```python
from build123d import *

# Parameters (mm, degrees)
F0_W     = 30
F0_H     = 20
F1_DEPTH = 7
F2_R     = 1.25
F3_DEPTH = 4
F4_W     = 30
F4_H     = 9
F5_DEPTH = 4


with BuildPart() as f1:
    # F0 (on Top) → F1 (new body)
    with BuildSketch(Plane.XY):
        Rectangle(F0_W, F0_H)
    extrude(amount=F1_DEPTH)

    # F2 (on face) → F3 (cut)
    with BuildSketch(Plane.XY.offset(7)):
        with Locations((5, 7.5)):
            Circle(F2_R)
        with Locations((-5, 7.5)):
            Circle(F2_R)
        with Locations((-5, -7.5)):
            Circle(F2_R)
        with Locations((5, -7.5)):
            Circle(F2_R)
    extrude(amount=-F3_DEPTH, mode=Mode.SUBTRACT)

    # F4 (on face) → F5 (cut)
    with BuildSketch(Plane(origin=(0, 0, 0), x_dir=(1, 0, 0), z_dir=(0, 0, -1))):
        Rectangle(F4_W, F4_H)
    extrude(amount=-F5_DEPTH, mode=Mode.SUBTRACT)


solid = f1.part
```
The listing builds one solid part. Answer for the finished solid, in the listing's coordinates (mm). A direction names the side the tool comes from. Coordinates: 2 decimals unless noted, no trailing zeros. Loops run counter-clockwise (first coordinate to the right, second up) from the corner with the lowest first, then second, coordinate; pieces in that order, holes last. Notation, with made-up numbers: (30.5, -15) -> (86.5, -15) arc R18 ccw to (86.5, -9) -> close; hole circle Ø9 at (-35.5, 47.5). An arc over 180 degrees is marked (long way). Return JSON: item names as keys, results as strings. Group by question number.
(1) Find the intervals of material crossed by probe 1 along Y at (x, z) = (5, 5.5); probe 2 along Y at (x, z) = (4.5, 6); probe 3 along Y at (x, z) = (5, 3.8), in increasing order. Write a range as from..to.
(2) Given pin 1 Ø0.8 at (x, y) = (-4.5, 7.5) entering from +Z; pin 2 Ø1 at (x, y) = (8.5, -1) entering from -Z, each flat-ended and moving along its own axis, determine where each tip first touches the part or whether it passes through.
(3) A cutting plane is placed at A-A on z = 5.25. Write down the section's boundary in (x, y).
(4) A cutting plane is placed at C-C on x = 0.5. Write down the section's boundary in (y, z).
(5) Which of the six approach directions +Z, -Z, +X, -X, +Y, -Y give full straight-line access (tool end or side, diameter ignored) to faces 5 (the flat face through (0, 0, 7)), 6 (the flat face through (5, -7, 3)), 7 (the flat face through (0, 0, 4))?
(6) Determine the mould class of faces 1 (the flat face through (0, -7, 0)), 2 (the flat face through (-5, 8, 3)), 3 (the flat face through (0, -10, 3)), 4 (the cylindrical face through (-5.27, -8.72, 5.03)) for opening direction Y: released by +Y, released by -Y, zero draft, split by the parting line, or undercut.
(7) A cutting plane is placed at D-D on z = 1.75. Write down the section's boundary in (x, y).
(8) A cutting plane is placed at B-B on z = 3.5. Write down the section's boundary in (x, y).
The answers:
{
 "1": {"probe 1": "y = -10..-8.75, -6.25..6.25, 8.75..10", "probe 2": "y = -10..-8.65, -6.35..6.35, 8.65..10", "probe 3": "y = -10..-8.75, -6.25..-4.5, 4.5..6.25, 8.75..10"},
 "2": {"pin 1": "stops at z = 3", "pin 2": "stops at z = 4"},
 "3": {"outline": "(-15, -10) -> (15, -10) -> (15, 10) -> (-15, 10) -> close; hole circle Ø2.5 at (-5, -7.5); hole circle Ø2.5 at (-5, 7.5); hole circle Ø2.5 at (5, -7.5); hole circle Ø2.5 at (5, 7.5)"},
 "4": {"outline": "(-10, 0) -> (-4.5, 0) -> (-4.5, 4) -> (4.5, 4) -> (4.5, 0) -> (10, 0) -> (10, 7) -> (-10, 7) -> close"},
 "5": {"face 5": "+Z, +X, -X, +Y, -Y", "face 6": "+Z", "face 7": "-Z, +X, -X"},
 "6": {"face 1": "zero draft", "face 2": "undercut", "face 3": "released by -Y", "face 4": "undercut"},
 "7": {"outline": "(-15, -10) -> (15, -10) -> (15, -4.5) -> (-15, -4.5) -> close; (-15, 4.5) -> (15, 4.5) -> (15, 10) -> (-15, 10) -> close"},
 "8": {"outline": "(-15, -10) -> (15, -10) -> (15, -4.5) -> (-15, -4.5) -> close; (-15, 4.5) -> (15, 4.5) -> (15, 10) -> (-15, 10) -> close; hole circle Ø2.5 at (-5, -7.5); hole circle Ø2.5 at (-5, 7.5); hole circle Ø2.5 at (5, -7.5); hole circle Ø2.5 at (5, 7.5)"}
}
